```python
from build123d import *

# Parameters (mm, degrees)
SKETCH2_W           = 0.8
SKETCH2_H           = 1.2
CUT_EXTRUDE2_REACH  = 53.658
SKETCH3_W           = 16.5
SKETCH3_H           = 5
SKETCH4_W           = 7.62
SKETCH4_H           = 2.2
BOSS_EXTRUDE1_DEPTH = 4
SKETCH5_W           = 7.62
SKETCH5_H           = 1.1
BOSS_EXTRUDE2_DEPTH = 3


with BuildPart() as part:
    # Sketch2 → Revolve1 (revolve)
    with BuildSketch(Plane.XY, mode=Mode.PRIVATE) as revolve1_sk:
        Polygon((0, -2), (0, 0), (36.5, 0), (34.5, -2), align=None)
        with Locations((34.9, 0.6)):
            Rectangle(SKETCH2_W, SKETCH2_H)
    revolve(revolve1_sk.sketch.rotate(Axis((0, 31.706596317, 0), (0, -1, 0)), 90), axis=Axis((0, 31.706596317, 0), (0, -1, 0)))

    # Sketch3 → Cut-Extrude2 (cut, up to next)
    with BuildSketch(Plane(origin=(0, 0, 0), x_dir=(1, 0, 0), z_dir=(0, 1, 0)), mode=Mode.PRIVATE) as cut_extrude2_sk1:
        with Locations((0, 27.5)):
            Rectangle(SKETCH3_W, SKETCH3_H)
    cut_extrude2_tool1 = extrude(cut_extrude2_sk1.sketch, amount=-CUT_EXTRUDE2_REACH, mode=Mode.PRIVATE) & part.part
    add(cut_extrude2_tool1.solids().sort_by_distance((0, 0, -27.5))[0], mode=Mode.SUBTRACT)

    # Sketch4 → Boss-Extrude1 (add)
    with BuildSketch(Plane(origin=(0, 0, 0), x_dir=(1, 0, 0), z_dir=(0, 1, 0))):
        with Locations((-17.78, 13)):
            Rectangle(SKETCH4_W, SKETCH4_H)
        with Locations((15.24, 13)):
            Rectangle(SKETCH4_W, SKETCH4_H)
    extrude(amount=BOSS_EXTRUDE1_DEPTH)

    # Sketch5 → Boss-Extrude2 (add)
    with BuildSketch(Plane(origin=(0, 4, 0), x_dir=(1, 0, 0), z_dir=(0, 1, 0))):
        with Locations((-17.78, 13.55)):
            Rectangle(SKETCH5_W, SKETCH5_H)
        with Locations((15.24, 13.55)):
            Rectangle(SKETCH5_W, SKETCH5_H)
    extrude(amount=BOSS_EXTRUDE2_DEPTH)


solid = part.part
```
Part model, mm, in its own coordinate system. A direction names the side the tool comes from. Round coordinates to 2 decimals unless told otherwise and drop trailing zeros. Write each loop counter-clockwise with the first axis right and the second up, starting at its lowest first coordinate (ties: lowest second). Pieces come first, ordered by that corner, then holes. Notation, with made-up numbers: M 37.25,37.25 L 68.25,37.25 A22 cw 68.25,71.25 Z; hole C 16.5,56.25 d8. An arc over 180 degrees is marked long. One line per question, with ' | ' between items.
(1) Two-plate mould, pull along X, no slides. Class faces 4 (the face through (34.46, 0.61, -7.65)), 5 (the face through (8, 1.2, -34)), 6 (the face through (-1.517, 0.608, -34.467)): released by +X, released by -X, zero draft, split by the parting line, or undercut.
Answer key:
face 4: split by the parting line | face 5: zero draft | face 6: undercut
(2) 3-axis set-ups, long thin cutter, end or side, ignore diameter. For faces 1 (the face through (0, -1, -25)), 2 (the face through (15, 5, -13)), 3 (the face through (-18, 2, -11.9)): which of +Z, -Z, +X, -X, +Y, -Y reach the whole face in a straight line?
Answer key:
face 1: +Y, -Y | face 2: +Z, +X, -X, +Y | face 3: +Y
(3) Saw through at C-C on z = 0. Write the cut outline in (x, y).
Answer key:
outline: M -36.5,0 L -34.5,-2 L 34.5,-2 L 36.5,0 L 35.3,0 L 35.3,1.2 L 34.5,1.2 L 34.5,0 L -34.5,0 L -34.5,1.2 L -35.3,1.2 L -35.3,0 Z
(4) Probe line 1 along Y through (x, z) = (21, -4); line 2 along X through (y, z) = (0.6, 0); line 3 along Z through (x, y) = (13, 5). List the from-to ranges inside material, lowest first.
Answer key:
line 1: y = -2 to 0 | line 2: x = -35.3 to -34.5, 34.5 to 35.3 | line 3: z = -14.1 to -13
(5) Saw through at A-A on x = 0. Write the cut outline in (y, z), then the cut area to 3 significant figures.
Answer key:
outline: M -2,-34.5 L 0,-36.5 L 0,-35.3 L 1.2,-35.3 L 1.2,-34.5 L 0,-34.5 L 0,-30 L -2,-30 Z; M -2,-25 L 0,-25 L 0,34.5 L 1.2,34.5 L 1.2,35.3 L 0,35.3 L 0,36.5 L -2,34.5 Z | area: 134 mm^2
(6) Saw through at B-B on y = 5.25. Write the cut outline in (x, z).
Answer key:
outline: M -21.59,-14.1 L -13.97,-14.1 L -13.97,-13 L -21.59,-13 Z; M 11.43,-14.1 L 19.05,-14.1 L 19.05,-13 L 11.43,-13 Z
(7) Pin check, flat tips, straight feed: pin 1 (0.6 mm diameter, centred on y = -1.5, z = -26.5, fed in from -X); pin 2 (1.2 mm diameter, centred on x = -18, y = 2, fed in from +Z); pin 3 (12 mm diameter, centred on x = -23.5, z = 29, fed in from -Y); pin 4 (2.5 mm diameter, centred on x = 15, y = 6, fed in from +Z). Stop position of each tip, or through.
Answer key:
pin 1: stops at x = -23.43 | pin 2: stops at z = -11.9 | pin 3: stops at y = -2 | pin 4: stops at z = -13
